Could you check a few things on this model? Use its own coordinates, in mm. Face numbers are marked on the shaded views. A direction names the side the tool comes from. Give positions to 0.01 mm unless a question says otherwise; leave off trailing zeros. Loops run counter-clockwise (first coordinate to the right, second up) from the corner with the lowest first, then second, coordinate; pieces in that order, holes last. Notation, with made-up numbers: (-36, 48) - (-23, 48) arc R22 ccw to (-23, 84) - close; hole circle Ø5 at (39, -29). An arc over 180 degrees is marked (long way). Write each question's results on one line, items separated by ' | '. Start each with the question number.
1) I want a section at A-A, the plane y = 9. Write out the boundary of the cut face in (x, z).
2) If we mould it in two halves opening along X, with no side actions, what happens to the marked faces 3 and 4? For each: +X half, -X half, draft (parallel to the pull), parting line (faces both ways), or undercut.
3) I want a section at C-C, the plane y = -44.5. Write out the boundary of the cut face in (x, z).
4) I want a section at B-B, the plane x = -73.5. Write out the boundary of the cut face in (y, z).
5) I'm going to push flat-ended pins straight in: pin 1 (0.5 mm diameter, centred on y = 35, z = 2.5, fed in from +X); pin 2 (10 mm diameter, centred on x = -85, y = -49.5, fed in from -Z); pin 3 (1 mm diameter, centred on x = -139.5, y = -33, fed in from -Z). Where does each tip first touch, or does it pass through?
6) I want a section at D-D, the plane x = -148. Write out the boundary of the cut face in (y, z), and give its area (3 significant figures).
7) On a 3-axis mill with a long thin cutter (end or side, diameter ignored), from which of +Z, -Z, +X, -X, +Y, -Y can I reach the whole of each face in a straight line? I mean the marked faces 1 and 2. Say none if no direction works.
8) If I drill on probe 1 along X at (y, z) = (-1, 1.45); probe 2 along Y at (x, z) = (93, -1.8); probe 3 along Z at (x, y) = (92.5, -65), over which ranges is the centre line in solid material (lowest first)? Write a range as [from, to].
from build123d import *

# Parameters (mm, degrees)
F0_W     = 221.5
F0_H     = 162
F1_DEPTH = 1
F0_W_2   = 225.5
F0_H_2   = 166
F2_DEPTH = 2
F3_DEPTH = 3
F4_DEPTH = 2


with BuildPart() as f1:
    # F0 (on Top) → F1 (new body, symmetric)
    with BuildSketch(Plane.XY):
        Rectangle(F0_W, F0_H)
    extrude(amount=F1_DEPTH, both=True)

    # F0 (on Top) → F2 (join, symmetric)
    with BuildSketch(Plane.XY):
        Rectangle(F0_W_2, F0_H_2)
        Rectangle(F0_W, F0_H, mode=Mode.SUBTRACT)
    extrude(amount=F2_DEPTH, both=True)

    # F0 (on Top) → F3 (join, symmetric)
    with BuildSketch(Plane.XY):
        Polygon((-112.75, -83), (-112.75, 83), (-117.75, 83), (-117.75, 50), (-117.75, -50), (-117.75, -83), align=None)
    extrude(amount=F3_DEPTH, both=True)

    # F0 (on Top) → F4 (join, symmetric)
    with BuildSketch(Plane.XY):
        Polygon((-117.75, -50), (-117.75, 50), (-217.25, 25), (-217.25, -25), align=None)
        Polygon((-182.25, -23.483152), (-207.25, -17.201745), (-207.25, 17.201745), (-182.25, 23.483152), align=None, mode=Mode.SUBTRACT)
    extrude(amount=F4_DEPTH, both=True)


solid = f1.part
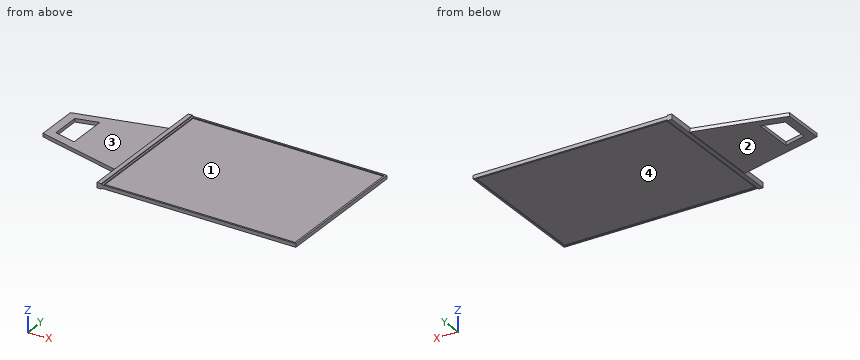
Answers:
1) outline: (-217.25, -2) - (-207.25, -2) - (-207.25, 2) - (-217.25, 2) - close; (-182.25, -2) - (-117.75, -2) - (-117.75, -3) - (-112.75, -3) - (-112.75, -2) - (-110.75, -2) - (-110.75, -1) - (110.75, -1) - (110.75, -2) - (112.75, -2) - (112.75, 2) - (110.75, 2) - (110.75, 1) - (-110.75, 1) - (-110.75, 2) - (-112.75, 2) - (-112.75, 3) - (-117.75, 3) - (-117.75, 2) - (-182.25, 2) - close
2) face 3: draft | face 4: undercut
3) outline: (-139.64, -2) - (-117.75, -2) - (-117.75, -3) - (-112.75, -3) - (-112.75, -2) - (-110.75, -2) - (-110.75, -1) - (110.75, -1) - (110.75, -2) - (112.75, -2) - (112.75, 2) - (110.75, 2) - (110.75, 1) - (-110.75, 1) - (-110.75, 2) - (-112.75, 2) - (-112.75, 3) - (-117.75, 3) - (-117.75, 2) - (-139.64, 2) - close
4) outline: (-83, -2) - (-81, -2) - (-81, -1) - (81, -1) - (81, -2) - (83, -2) - (83, 2) - (81, 2) - (81, 1) - (-81, 1) - (-81, 2) - (-83, 2) - close
5) pin 1: stops at x = -112.75 | pin 2: stops at z = -1 | pin 3: stops at z = -2
6) outline: (-42.4, -2) - (42.4, -2) - (42.4, 2) - (-42.4, 2) - close | area: 339 mm2
7) face 1: +Z | face 2: -Z, -X, +Y, -Y
8) probe 1: x = [-217.25, -207.25], [-182.25, -110.75], [110.75, 112.75] | probe 2: y = [-83, -81], [81, 83] | probe 3: z = [-1, 1]
